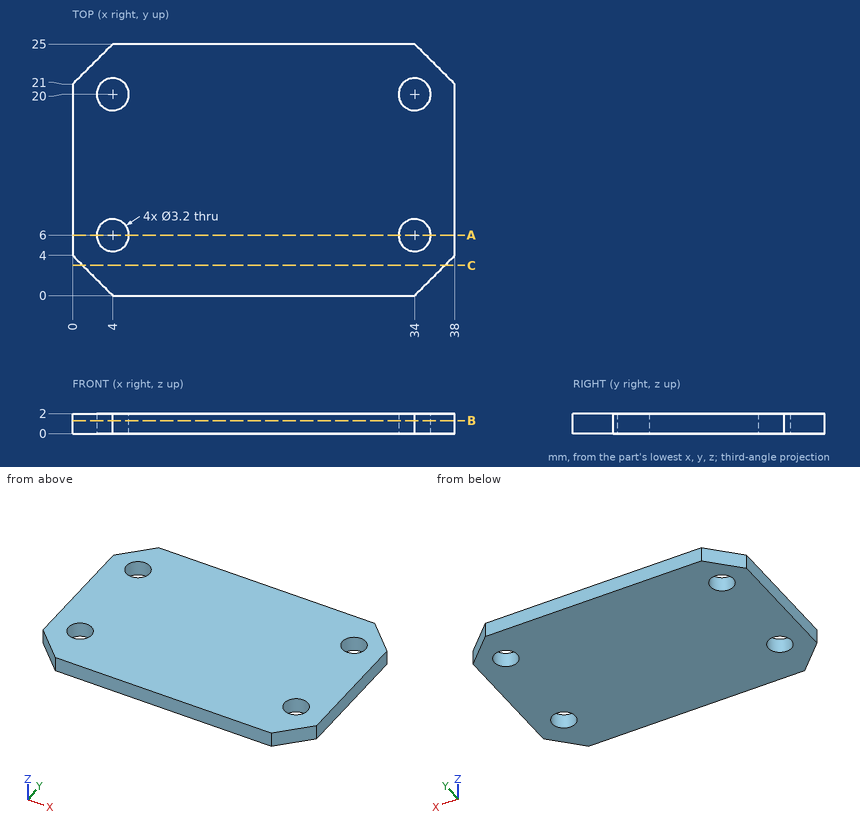
Verification items for this drawing (mm, ordinates from the low corner). Coordinates: 2 decimals unless noted, no trailing zeros. Write each loop counter-clockwise with the first axis right and the second up, starting at its lowest first coordinate (ties: lowest second). Pieces come first, ordered by that corner, then holes. Notation, with made-up numbers: M -2.5,-35.5 L 15.5,-35.5 A11 ccw 15.5,-29.5 Z; hole C -15.75,34 d10. An arc over 180 degrees is marked long. Answer as a JSON object with one key per item and string values. Group by question number.
(1) Gauge pin test, flat end, axial feed: pin 1 (2.5 mm diameter, centred on x = 4, y = 6, fed in from -Z). Record the tip position at first contact, or that the pin passes through.
(2) Cross-section at A-A, the plane y = 6. Record the cut outline in (x, z), and give its area (3 significant figures).
(3) Material ranges on line 1 (Y direction, x = 4, z = 0.5); line 2 (Y direction, x = 4.5, z = 1.7); line 3 (X direction, y = 5, z = 1.4), recorded low to high.
(4) Cross-section at C-C, the plane y = 3. Record the cut outline in (x, z).
(5) Cross-section at B-B, the plane z = 1.3. Record the cut outline in (x, y).
Reply:
{
 "1": {"pin 1": "through"},
 "2": {"outline": "M 0,0 L 2.4,0 L 2.4,2 L 0,2 Z; M 5.6,0 L 32.4,0 L 32.4,2 L 5.6,2 Z; M 35.6,0 L 38,0 L 38,2 L 35.6,2 Z", "area": "63.2 mm²"},
 "3": {"line 1": "0 to 4.4, 7.6 to 18.4, 21.6 to 25", "line 2": "0 to 4.48, 7.52 to 18.48, 21.52 to 25", "line 3": "0 to 2.75, 5.25 to 32.75, 35.25 to 38"},
 "4": {"outline": "M 1,0 L 37,0 L 37,2 L 1,2 Z"},
 "5": {"outline": "M 0,4 L 4,0 L 34,0 L 38,4 L 38,21 L 34,25 L 4,25 L 0,21 Z; hole C 4,6 d3.2; hole C 4,20 d3.2; hole C 34,6 d3.2; hole C 34,20 d3.2"}
}
